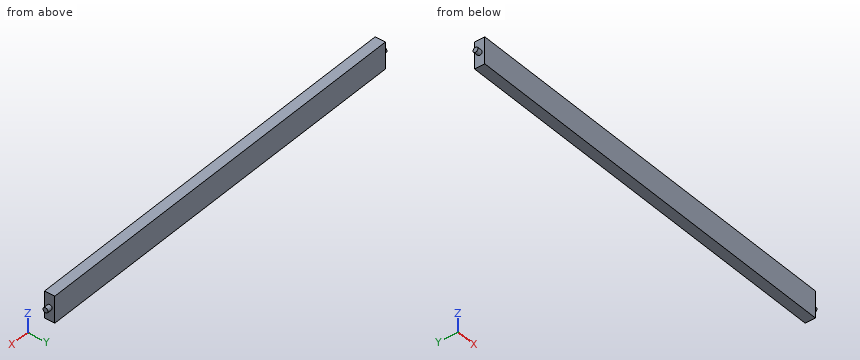
```python
from build123d import *

# Parameters (mm, degrees)
F0_W     = 755.65
F0_H     = 19.05
F1_DEPTH = 50.8
F3_R     = 4.7625
F4_DEPTH = 9.525
F6_R     = 4.7625
F7_DEPTH = 9.525


with BuildPart() as f1:
    # F0 (on Top) → F1 (new body)
    with BuildSketch(Plane.XY):
        Rectangle(F0_W, F0_H)
    extrude(amount=F1_DEPTH)

    # F3 (on offset) → F4 (join)
    with BuildSketch(Plane.YZ.offset(377.825)):
        with Locations((0, 25.4)):
            Circle(F3_R)
    extrude(amount=F4_DEPTH)

    # F6 (on offset) → F7 (join)
    with BuildSketch(Plane.YZ.offset(-377.825)):
        with Locations((0, 25.418339)):
            Circle(F6_R)
    extrude(amount=-F7_DEPTH)


solid = f1.part
```
Model file for the job. Use its own axes, mm. Coordinates: 2 decimals unless noted, no trailing zeros. Write each loop counter-clockwise with the first axis right and the second up, starting at its lowest first coordinate (ties: lowest second). Pieces come first, ordered by that corner, then holes. Notation, with made-up numbers: (10, 62) - (32, 62) arc R13 ccw to (32, 73) - close; hole circle Ø8 at (-20.5, 58). An arc over 180 degrees is marked (long way). One line per item, written item: value. Start each with the question number.
1. Probe line 1 (X direction, y = 5, z = 9) (3 decimals). List the from-to ranges inside material, lowest first. Write a range as from..to.
2. Slice it at B-B (z = 14). Write the cut outline in (x, y) (3 decimals), plus the area to 3 significant figures.
3. Flat gauge pins, fed straight in: pin 1 (6 mm diameter, centred on y = -6, z = 43, fed in from -X) (3 decimals); pin 2 (8 mm diameter, centred on y = -1.5, z = 36, fed in from +X) (3 decimals). Where does each tip first touch, or does it go through?
Answers below:
1. line 1: x = -377.825..377.825
2. outline: (-377.825, -9.525) - (377.825, -9.525) - (377.825, 9.525) - (-377.825, 9.525) - close
2. area: 14,400 mm^2
3. pin 1: stops at x = -377.825
3. pin 2: stops at x = 377.825
